Verification items for the finished model (mm, model axes). Face numbers are marked on the shaded views. A direction names the side the tool comes from. Give positions to 0.01 mm unless a question says otherwise; leave off trailing zeros. Loops run counter-clockwise (first coordinate to the right, second up) from the corner with the lowest first, then second, coordinate; pieces in that order, holes last. Notation, with made-up numbers: M -24.5,75 L -13.5,75 A12 ccw -13.5,82 Z; hole C 0.25,12 d2. An arc over 180 degrees is marked long. Use a Markdown table: item, result.
from build123d import *

# Parameters (mm, degrees)
HOLE_WIZARD_M61_D           = 5
HOLE_WIZARD_M61_DEPTH       = 17
HOLE_WIZARD_M61_CSINK_D     = 7
HOLE_WIZARD_M61_CSINK_ANGLE = 90
HOLE_WIZARD_M61_TIP         = 1.502151548
HOLE_WIZARD_M62_D           = 5
HOLE_WIZARD_M62_DEPTH       = 17
HOLE_WIZARD_M62_CSINK_D     = 7
HOLE_WIZARD_M62_CSINK_ANGLE = 90
HOLE_WIZARD_M62_TIP         = 1.502151548
SKETCH_5_W                  = 1.2
SKETCH_5_H                  = 0.45
CHAMFER_2_SIZE              = 0.5


with BuildPart() as part:
    # Эскиз1 → Повернуть1 (revolve)
    with BuildSketch(Plane.XY, mode=Mode.PRIVATE) as revolve_1_sk:
        Polygon((-26.5, 0), (-26.5, 6), (-22.5, 6), (-22.5, 7.5), (22.5, 7.5), (22.5, 6), (26.5, 6), (26.5, 0), align=None)
    revolve(revolve_1_sk.sketch.rotate(Axis((0, 0, 0), (-1, 0, 0)), 90), axis=Axis((0, 0, 0), (-1, 0, 0)))

    # Отверстие обработанное метчиком M61
    with Locations(Plane.ZY.offset(26.5)):
        with Locations((0, 0)):
            CounterSinkHole(HOLE_WIZARD_M61_D / 2, HOLE_WIZARD_M61_CSINK_D / 2, depth=HOLE_WIZARD_M61_DEPTH, counter_sink_angle=HOLE_WIZARD_M61_CSINK_ANGLE)
            with Locations((0, 0, -(HOLE_WIZARD_M61_DEPTH + HOLE_WIZARD_M61_TIP / 2))):  # 118° drill point
                Cone(0, HOLE_WIZARD_M61_D / 2, HOLE_WIZARD_M61_TIP, mode=Mode.SUBTRACT)

    # Отверстие обработанное метчиком M62
    with Locations(Plane(origin=(26.5, 0, 0), x_dir=(0, 0, -1), z_dir=(1, 0, 0))):
        with Locations((0, 0)):
            CounterSinkHole(HOLE_WIZARD_M62_D / 2, HOLE_WIZARD_M62_CSINK_D / 2, depth=HOLE_WIZARD_M62_DEPTH, counter_sink_angle=HOLE_WIZARD_M62_CSINK_ANGLE)
            with Locations((0, 0, -(HOLE_WIZARD_M62_DEPTH + HOLE_WIZARD_M62_TIP / 2))):  # 118° drill point
                Cone(0, HOLE_WIZARD_M62_D / 2, HOLE_WIZARD_M62_TIP, mode=Mode.SUBTRACT)

    # Эскиз5 → Вырез-Повернуть1 (revolve, cut)
    with BuildSketch(Plane.XY, mode=Mode.PRIVATE) as cut_revolve_1_sk:
        with Locations((-18.4, 7.275)):
            Rectangle(SKETCH_5_W, SKETCH_5_H)
        with Locations((18.4, 7.275)):
            Rectangle(SKETCH_5_W, SKETCH_5_H)
    revolve(cut_revolve_1_sk.sketch.rotate(Axis((0, 0, 0), (-1, 0, 0)), 90), axis=Axis((0, 0, 0), (-1, 0, 0)), mode=Mode.SUBTRACT)

    # Фаска2
    chamfer_2_edges = [part.edges().sort_by_distance(p)[0] for p in [
        (26.5, 0, 6),
        (22.5, 0, 7.5),
        (-22.5, 0, 7.5),
        (-26.5, 0, 6),
    ]]
    chamfer(chamfer_2_edges, length=CHAMFER_2_SIZE)


solid = part.part
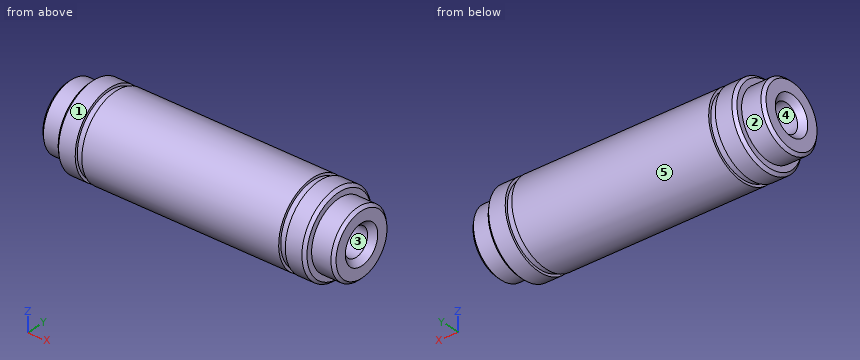
(1) Material ranges on line 1 (Y direction, x = 15.75, z = 0); line 2 (Z direction, x = 24.5, y = 1.75); line 3 (Y direction, x = 10, z = 0.75), recorded low to high.
Results below:
| item | result |
|---|---|
| line 1 | -7.5 to -2.5, 2.5 to 7.5 |
| line 2 | -5.74 to -1.79, 1.79 to 5.74 |
| line 3 | -7.46 to -2.38, 2.38 to 7.46 |
(2) Cross-section at A-A on x = -23. Record the cut outline in (y, z), then the cut area to 3 significant figures.
Results below:
| item | result |
|---|---|
| outline | C 0,0 d12; hole C 0,0 d5 |
| area | 93.5 mm^2 |
(3) Cross-section at B-B on x = 0.5. Record the cut outline in (y, z), then the cut area to 3 significant figures.
Results below:
| item | result |
|---|---|
| outline | C 0,0 d15 |
| area | 177 mm^2 |
(4) Gauge pin test, flat ends, axial feed: P1, Ø4, axis at y = 0, z = 0, coming from the -X side; P2, Ø2, axis at x = -7.5, y = -1.5, coming from the -Z side; P3, Ø1.5, axis at x = 12, z = -3, coming from the -Y side. Record the tip position at first contact, or that the pin passes through.
Results below:
| item | result |
|---|---|
| P1 | x = -9.2 |
| P2 | z = -7.48 |
| P3 | y = -7.15 |
(5) Draft check along Z on the marked faces 4 and 5. Enter one of: +Z half, -Z half, draft (parallel to the pull), parting line (faces both ways), or undercut.
Results below:
| item | result |
|---|---|
| face 4 | undercut |
| face 5 | parting line |
(6) Set-up check for the marked faces 1, 2 and 3: record each of +Z, -Z, +X, -X, +Y, -Y from which the full face is reachable in a straight line by a thin tool's end or side.
Results below:
| item | result |
|---|---|
| face 1 | +X, -X |
| face 2 | -X |
| face 3 | +X |
